CAD build for the part. Positions are in the model's coordinates, mm. Face numbers are marked on the shaded views. Round coordinates to 2 decimals unless told otherwise and drop trailing zeros.
from build123d import *

# Parameters (mm, degrees)
BOSS_EXTRU_1_DEPTH = 1
CONG_1_R           = 1


with BuildPart() as part:
    # Esquisse1 → Révolution1 (revolve)
    with BuildSketch(Plane(origin=(0, 0, 0), x_dir=(0, 0, -1), z_dir=(1, 0, 0)), mode=Mode.PRIVATE) as r_volution1_sk:
        Polygon((3, 9), (3, 8.3), (3.8, 8.3), (3.8, 9), (4.6, 9), (4.6, 8.3), (5.4, 8.3), (5.4, 9), (6.2, 9), (6.2, 8.3), (7, 8.3), (7, 9), (7.8, 9), (7.8, 8.3), (8.6, 8.3), (8.6, 9), (9.4, 9), (9.4, 8.3), (10.2, 8.3), (10.2, 9), (11, 9), (11, 8.3), (11.8, 8.3), (11.8, 9), (12.6, 9), (12.6, 8.3), (13.4, 8.3), (13.4, 9), (14.2, 9), (14.2, 8.3), (15, 8.3), (15, 9), (15.8, 9), (15.8, 8.3), (16.6, 8.3), (16.6, 9), (17.4, 9), (17.4, 8.3), (18.2, 8.3), (18.2, 9), (19, 9), (19, 8.3), (19.8, 8.3), (19.8, 9), (20.6, 9), (20.6, 8.3), (21.4, 8.3), (21.4, 9), (22.2, 9), (22.2, 8.3), (23, 8.3), (23, 9), (23.8, 9), (23.8, 8.3), (24.6, 8.3), (24.6, 9), (25.4, 9), (25.4, 8.3), (26.2, 8.3), (26.2, 9), (27, 9), (27, 8.3), (27.8, 8.3), (27.8, 9), (28.6, 9), (28.6, 8.3), (29.4, 8.3), (29.4, 9), (30.2, 9), (30.2, 8.3), (31, 8.3), (31, 9), (31.8, 9), (31.8, 8.3), (32.6, 8.3), (32.6, 9), (33.4, 9), (33.4, 8.3), (34.2, 8.3), (34.2, 9), (35, 9), (35, 8.3), (35.8, 8.3), (35.8, 9), (36.6, 9), (36.6, 8.3), (37.4, 8.3), (37.4, 9), (38.2, 9), (38.2, 8.3), (39, 8.3), (39, 9), (39.8, 9), (39.8, 8.3), (40.6, 8.3), (40.6, 9), (41.4, 9), (41.4, 8.3), (42.2, 8.3), (42.2, 9), (44, 9), (44, 0), (1, 0), (1, 7.5), (0, 7.5), (0, 9), (2, 9), (2, 8.8), (2.2, 8.8), (2.2, 9), align=None)
    revolve(r_volution1_sk.sketch.rotate(Axis((0, 0, -1), (0, 0, -1)), 90), axis=Axis((0, 0, -1), (0, 0, -1)))

    # Esquisse2 → Boss.-Extru.1 (add)
    with BuildSketch(Plane.XY.offset(-1)):
        with BuildLine():
            Line((-1.5, 4.5), (1.5, 4.5))
            ThreePointArc((1.5, 4.5), (2.207106781, 4.207106781), (2.5, 3.5))
            Line((2.5, 3.5), (2.5, 2.5))
            ThreePointArc((2.5, 2.5), (2.207106781, 1.792893219), (1.5, 1.5))
            Line((1.5, 1.5), (-1.5, 1.5))
            ThreePointArc((-1.5, 1.5), (-2.207106781, 1.792893219), (-2.5, 2.5))
            Line((-2.5, 2.5), (-2.5, 3.5))
            ThreePointArc((-2.5, 3.5), (-2.207106781, 4.207106781), (-1.5, 4.5))
        make_face()
        with BuildLine():
            Line((1.5, -1.5), (-1.5, -1.5))
            ThreePointArc((-1.5, -1.5), (-2.207106781, -1.792893219), (-2.5, -2.5))
            Line((-2.5, -2.5), (-2.5, -3.5))
            ThreePointArc((-2.5, -3.5), (-2.207106781, -4.207106781), (-1.5, -4.5))
            Line((-1.5, -4.5), (1.5, -4.5))
            ThreePointArc((1.5, -4.5), (2.207106781, -4.207106781), (2.5, -3.5))
            Line((2.5, -3.5), (2.5, -2.5))
            ThreePointArc((2.5, -2.5), (2.207106781, -1.792893219), (1.5, -1.5))
        make_face()
    extrude(amount=BOSS_EXTRU_1_DEPTH)

    # Congé1
    cong_1_edges = [part.edges().sort_by_distance(p)[0] for p in [
        (2.5, -3, 0),
        (2.207106781, -4.207106781, 0),
        (0, -4.5, 0),
        (-2.207106781, -4.207106781, 0),
        (-2.5, -3, 0),
        (-2.207106781, -1.792893219, 0),
        (0, -1.5, 0),
        (2.207106781, -1.792893219, 0),
        (2.5, 3, 0),
        (2.207106781, 1.792893219, 0),
        (0, 1.5, 0),
        (-2.207106781, 1.792893219, 0),
        (-2.5, 3, 0),
        (-2.207106781, 4.207106781, 0),
        (0, 4.5, 0),
        (2.207106781, 4.207106781, 0),
    ]]
    fillet(cong_1_edges, radius=CONG_1_R - 0.0001)  # a hair under: the kernel refuses the full size


solid = part.part
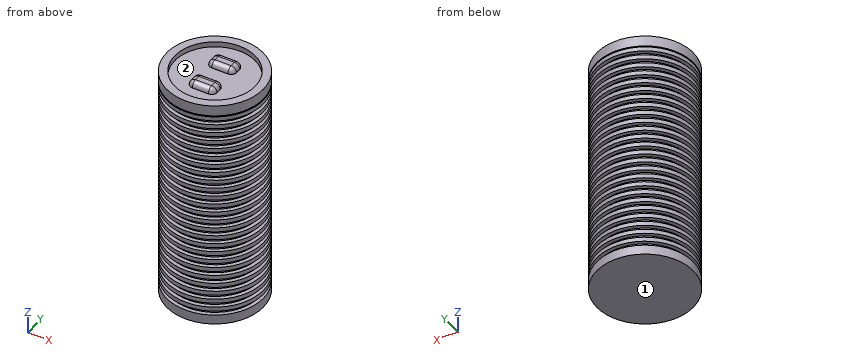
Item 1: Mould opens along Y. For the marked faces 1 and 2 say: released by +Y, released by -Y, zero draft, split by the parting line, or undercut.
Verdict:
face 1: zero draft
face 2: undercut
Item 2: Flat gauge pins, fed straight in: P1, Ø1, axis at y = -2, z = -5.5, coming from the +X side; P2, Ø1, axis at x = -4, z = -37, coming from the -Y side. Where does each tip first touch, or does it go through?
Verdict:
P1: stops at x = 8.87
P2: stops at y = -8.2
Item 3: Wall check: L1, parallel to Y at x = 0, z = -0.15; L2, parallel to Y at x = 0, z = -0.6; L3, parallel to Z at x = -2, y = 0.75. Give the ranges that are in metal, low to high.
Verdict:
L1: y = -9 to -7.5, -4.03 to -1.97, 1.97 to 4.03, 7.5 to 9
L2: y = -9 to -7.5, -4.42 to -1.58, 1.58 to 4.42, 7.5 to 9
L3: z = -44 to -1
